```python
from build123d import *

# Parameters (mm, degrees)
F0_R     = 16
F0_R_2   = 2.5
F1_DEPTH = 15
F2_DEPTH = 5
F3_R     = 5.5
F3_R_2   = 2.5
F4_DEPTH = 6.5


# Not quite as in the source:
# - a feature names something its author has since deleted; it is built from what else it names


with BuildPart() as f1:
    # F0 (on Front) → F1 (new body)
    with BuildSketch(Plane.XZ):
        with BuildLine():
            ThreePointArc((139.0482066844, -68.5256164076), (148.1685102123, -58.5964356365), (151.4733932528, -45.5256164076))
            ThreePointArc((151.4733932528, -45.5256164076), (110.9025740239, -21.3304994481), (108.8985798211, -68.5256164076))
            ThreePointArc((108.8985798211, -68.5256164076), (123.9733932528, -73.0256164076), (139.0482066844, -68.5256164076))
        make_face()
        with BuildLine():
            ThreePointArc((104.6679489936, -37.2612457748), (103.6217962638, -33.7756164076), (107.1635162088, -32.9387965643))
            ThreePointArc((107.1635162088, -32.9387965643), (123.9733932528, -24.5256164076), (140.7832702967, -32.9387965643))
            ThreePointArc((140.7832702967, -32.9387965643), (143.344907515, -32.8242939541), (144.6599267322, -35.0256164076))
            ThreePointArc((144.6599267322, -35.0256164076), (144.2868114199, -36.3395271829), (143.2788375119, -37.2612457748))
            ThreePointArc((143.2788375119, -37.2612457748), (144.5453927842, -41.307460972), (144.9733932528, -45.5256164076))
            ThreePointArc((144.9733932528, -45.5256164076), (139.6801897358, -59.4646459377), (126.468960468, -66.3768068838))
            ThreePointArc((126.468960468, -66.3768068838), (126.4722848108, -66.4511786418), (126.4733932528, -66.5256164076))
            ThreePointArc((126.4733932528, -66.5256164076), (123.8989554869, -69.0245079657), (121.4778260376, -66.3768068838))
            ThreePointArc((121.4778260376, -66.3768068838), (105.7868597733, -56.0256164076), (104.6679489936, -37.2612457748))
        make_face(mode=Mode.SUBTRACT)
        with BuildLine():
            ThreePointArc((107.1635162088, -32.9387965643), (107.9881822268, -33.8406356249), (108.2868597733, -35.0256164076))
            ThreePointArc((108.2868597733, -35.0256164076), (107.1007705486, -37.1525010953), (104.6679489936, -37.2612457748))
            ThreePointArc((104.6679489936, -37.2612457748), (105.7868597733, -56.0256164076), (121.4778260376, -66.3768068838))
            ThreePointArc((121.4778260376, -66.3768068838), (123.9733932528, -64.0256164076), (126.468960468, -66.3768068838))
            ThreePointArc((126.468960468, -66.3768068838), (139.6801897358, -59.4646459377), (144.9733932528, -45.5256164076))
            ThreePointArc((144.9733932528, -45.5256164076), (144.5453927842, -41.307460972), (143.2788375119, -37.2612457748))
            ThreePointArc((143.2788375119, -37.2612457748), (139.9948632228, -36.2756164076), (140.7832702967, -32.9387965643))
            ThreePointArc((140.7832702967, -32.9387965643), (123.9733932528, -24.5256164076), (107.1635162088, -32.9387965643))
        make_face()
        with Locations((123.9733932528, -45.5256164076)):
            Circle(F0_R, mode=Mode.SUBTRACT)
        with BuildLine():
            ThreePointArc((108.8985798211, -68.5256164076), (110.9025740239, -21.3304994481), (151.4733932528, -45.5256164076))
            ThreePointArc((151.4733932528, -45.5256164076), (148.1685102123, -58.5964356365), (139.0482066844, -68.5256164076))
            Line((139.0482066844, -68.5256164076), (207.9733932528, -68.5256164076))
            Line((207.9733932528, -68.5256164076), (207.9733932528, 11.3154806698))
            Line((207.9733932528, 11.3154806698), (39.9733932528, 11.3154806698))
            Line((39.9733932528, 11.3154806698), (39.9733932528, -68.5256164076))
            Line((39.9733932528, -68.5256164076), (108.8985798211, -68.5256164076))
        make_face()
        with BuildLine():
            ThreePointArc((139.0482066844, -68.5256164076), (123.9733932528, -73.0256164076), (108.8985798211, -68.5256164076))
            Line((108.8985798211, -68.5256164076), (39.9733932528, -68.5256164076))
            Line((39.9733932528, -68.5256164076), (39.9733932528, -88.8428396075))
            Line((39.9733932528, -88.8428396075), (207.9733932528, -88.8428396075))
            Line((207.9733932528, -88.8428396075), (207.9733932528, -68.5256164076))
            Line((207.9733932528, -68.5256164076), (139.0482066844, -68.5256164076))
        make_face()
        with Locations((48.9733932528, -76.0256164076)):
            Circle(F0_R_2, mode=Mode.SUBTRACT)
        with Locations((78.9733932528, -76.0256164076)):
            Circle(F0_R_2, mode=Mode.SUBTRACT)
        with Locations((108.9733932528, -76.0256164076)):
            Circle(F0_R_2, mode=Mode.SUBTRACT)
        with Locations((138.9733932528, -76.0256164076)):
            Circle(F0_R_2, mode=Mode.SUBTRACT)
        with Locations((168.9733932528, -76.0256164076)):
            Circle(F0_R_2, mode=Mode.SUBTRACT)
        with Locations((198.9733932528, -76.0256164076)):
            Circle(F0_R_2, mode=Mode.SUBTRACT)
    extrude(amount=F1_DEPTH)

    # F0 (on Front) → F2 (cut)
    with BuildSketch(Plane.XZ):
        with BuildLine():
            ThreePointArc((139.0482066844, -68.5256164076), (148.1685102123, -58.5964356365), (151.4733932528, -45.5256164076))
            ThreePointArc((151.4733932528, -45.5256164076), (110.9025740239, -21.3304994481), (108.8985798211, -68.5256164076))
            ThreePointArc((108.8985798211, -68.5256164076), (123.9733932528, -73.0256164076), (139.0482066844, -68.5256164076))
        make_face()
        with BuildLine():
            ThreePointArc((104.6679489936, -37.2612457748), (103.6217962638, -33.7756164076), (107.1635162088, -32.9387965643))
            ThreePointArc((107.1635162088, -32.9387965643), (123.9733932528, -24.5256164076), (140.7832702967, -32.9387965643))
            ThreePointArc((140.7832702967, -32.9387965643), (143.344907515, -32.8242939541), (144.6599267322, -35.0256164076))
            ThreePointArc((144.6599267322, -35.0256164076), (144.2868114199, -36.3395271829), (143.2788375119, -37.2612457748))
            ThreePointArc((143.2788375119, -37.2612457748), (144.5453927842, -41.307460972), (144.9733932528, -45.5256164076))
            ThreePointArc((144.9733932528, -45.5256164076), (139.6801897358, -59.4646459377), (126.468960468, -66.3768068838))
            ThreePointArc((126.468960468, -66.3768068838), (126.4722848108, -66.4511786418), (126.4733932528, -66.5256164076))
            ThreePointArc((126.4733932528, -66.5256164076), (123.8989554869, -69.0245079657), (121.4778260376, -66.3768068838))
            ThreePointArc((121.4778260376, -66.3768068838), (105.7868597733, -56.0256164076), (104.6679489936, -37.2612457748))
        make_face(mode=Mode.SUBTRACT)
        with BuildLine():
            ThreePointArc((107.1635162088, -32.9387965643), (107.9881822268, -33.8406356249), (108.2868597733, -35.0256164076))
            ThreePointArc((108.2868597733, -35.0256164076), (107.1007705486, -37.1525010953), (104.6679489936, -37.2612457748))
            ThreePointArc((104.6679489936, -37.2612457748), (105.7868597733, -56.0256164076), (121.4778260376, -66.3768068838))
            ThreePointArc((121.4778260376, -66.3768068838), (123.9733932528, -64.0256164076), (126.468960468, -66.3768068838))
            ThreePointArc((126.468960468, -66.3768068838), (139.6801897358, -59.4646459377), (144.9733932528, -45.5256164076))
            ThreePointArc((144.9733932528, -45.5256164076), (144.5453927842, -41.307460972), (143.2788375119, -37.2612457748))
            ThreePointArc((143.2788375119, -37.2612457748), (139.9948632228, -36.2756164076), (140.7832702967, -32.9387965643))
            ThreePointArc((140.7832702967, -32.9387965643), (123.9733932528, -24.5256164076), (107.1635162088, -32.9387965643))
        make_face()
        with Locations((123.9733932528, -45.5256164076)):
            Circle(F0_R, mode=Mode.SUBTRACT)
        with BuildLine():
            ThreePointArc((139.0482066844, -68.5256164076), (123.9733932528, -73.0256164076), (108.8985798211, -68.5256164076))
            Line((108.8985798211, -68.5256164076), (39.9733932528, -68.5256164076))
            Line((39.9733932528, -68.5256164076), (39.9733932528, -88.8428396075))
            Line((39.9733932528, -88.8428396075), (207.9733932528, -88.8428396075))
            Line((207.9733932528, -88.8428396075), (207.9733932528, -68.5256164076))
            Line((207.9733932528, -68.5256164076), (139.0482066844, -68.5256164076))
        make_face()
        with Locations((48.9733932528, -76.0256164076)):
            Circle(F0_R_2, mode=Mode.SUBTRACT)
        with Locations((78.9733932528, -76.0256164076)):
            Circle(F0_R_2, mode=Mode.SUBTRACT)
        with Locations((108.9733932528, -76.0256164076)):
            Circle(F0_R_2, mode=Mode.SUBTRACT)
        with Locations((138.9733932528, -76.0256164076)):
            Circle(F0_R_2, mode=Mode.SUBTRACT)
        with Locations((168.9733932528, -76.0256164076)):
            Circle(F0_R_2, mode=Mode.SUBTRACT)
        with Locations((198.9733932528, -76.0256164076)):
            Circle(F0_R_2, mode=Mode.SUBTRACT)
    extrude(amount=F2_DEPTH, mode=Mode.SUBTRACT)

    # F3 (on face) → F4 (cut)
    with BuildSketch(Plane.XZ.offset(15)):
        with Locations((198.9733932528, -76.0256164076)):
            Circle(F3_R)
        with Locations((198.9733932528, -76.0256164076)):
            Circle(F3_R_2, mode=Mode.SUBTRACT)
        with Locations((168.9733932528, -76.0256164076)):
            Circle(F3_R)
        with Locations((168.9733932528, -76.0256164076)):
            Circle(F3_R_2, mode=Mode.SUBTRACT)
        with Locations((138.9733932528, -76.0256164076)):
            Circle(F3_R)
        with Locations((138.9733932528, -76.0256164076)):
            Circle(F3_R_2, mode=Mode.SUBTRACT)
        with Locations((108.9733932528, -76.0256164076)):
            Circle(F3_R)
        with Locations((108.9733932528, -76.0256164076)):
            Circle(F3_R_2, mode=Mode.SUBTRACT)
        with Locations((78.9733932528, -76.0256164076)):
            Circle(F3_R)
        with Locations((78.9733932528, -76.0256164076)):
            Circle(F3_R_2, mode=Mode.SUBTRACT)
        with Locations((48.9733932528, -76.0256164076)):
            Circle(F3_R)
        with Locations((48.9733932528, -76.0256164076)):
            Circle(F3_R_2, mode=Mode.SUBTRACT)
    extrude(amount=-F4_DEPTH, mode=Mode.SUBTRACT)


solid = f1.part
```
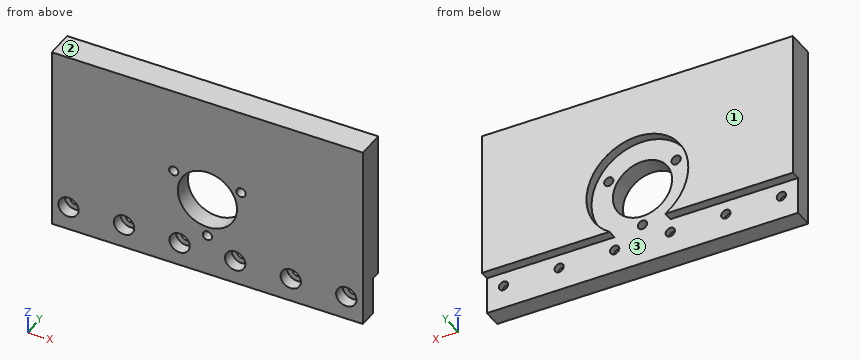
The model under review builds one solid part; all positions refer to its coordinate system, in mm. Face numbers are marked on the shaded views. Round coordinates to 2 decimals unless told otherwise and drop trailing zeros. Write each loop counter-clockwise with the first axis right and the second up, starting at its lowest first coordinate (ties: lowest second). Pieces come first, ordered by that corner, then holes.
(1) We need section D-D on z = -27. Give the boundary of the cut face in (x, y).
(2) Wall thickness on L1, parallel to X at y = -6.5, z = -46; L2, parallel to X at y = -5.75, z = -48.5; L3, parallel to Z at x = 123, y = -11: over which ranges is each line inside the solid? List them lowest first.
(3) Insertion check: pin 1 (2 mm diameter, centred on x = 118.5, z = -57.5, fed in from +Y) (3 decimals); pin 2 (6.5 mm diameter, centred on x = 138.97, z = -76.03, fed in from -Y); pin 3 (6 mm diameter, centred on x = 168.97, z = -76.03, fed in from +Y). Each pin has a flat end and moves straight along its axis. Give the tip position at first contact, or say it passes through.
(4) We need section A-A on x = 169.5. Give the boundary of the cut face in (y, z), and give its area (3 significant figures).
(5) We need section C-C on y = -13. Give the number of separate pieces and of enclosed holes in the cut face, and give its area (3 significant figures).
(6) We need section B-B on z = -48.5. Give the boundary of the cut face in (x, y).
(7) Mouldability with a two-part tool opening along Z and no side actions: class the marked faces 1, 2 and 3 as +Z half, -Z half, draft (parallel to the pull), parting line (faces both ways), or undercut.
Findings below:
1. outline: (39.97, -15) - (207.97, -15) - (207.97, 0) - (144.3, 0) - (144.3, -5) - (103.65, -5) - (103.65, 0) - (39.97, 0) - close
2. L1: x = 39.97 to 107.98, 139.97 to 207.97
2. L2: x = 39.97 to 108.25, 139.69 to 207.97
2. L3: z = -88.84 to -68.83, -64.22 to -61.5, -29.56 to 11.32
3. pin 1: passes through
3. pin 2: stops at y = -8.5
3. pin 3: stops at y = -5
4. outline: (-15, -88.84) - (-5, -88.84) - (-5, -78.47) - (-8.5, -78.47) - (-8.5, -81.5) - (-15, -81.5) - close; (-15, -70.55) - (-8.5, -70.55) - (-8.5, -73.58) - (-5, -73.58) - (-5, -68.53) - (0, -68.53) - (0, 11.32) - (-15, 11.32) - close
4. area: 1,310 mm2
5. separate pieces: 1
5. enclosed holes: 10
5. area: 15,400 mm2
6. outline: (39.97, -15) - (108.25, -15) - (108.25, -5) - (96.63, -5) - (96.63, 0) - (39.97, 0) - close; (139.69, -15) - (207.97, -15) - (207.97, 0) - (151.31, 0) - (151.31, -5) - (139.69, -5) - close
7. face 1: draft
7. face 2: +Z half
7. face 3: undercut
